```python
from build123d import *

# Parameters (mm, degrees)
BASE_FLANGE1_DEPTH = 390.5
CUT_EXTRUDE2_DEPTH = 419.369827425


# Sheet-metal steps are written as plain solids
with BuildPart() as part:
    # Sketch1 → Base-Flange1 (new, symmetric)
    with BuildSketch(Plane(origin=(0, 0, 0), x_dir=(1, 0, 0), z_dir=(0, 1, 0))):
        with BuildLine():
            Line((9.5, 58), (9.5, 68.0134))
            ThreePointArc((9.5, 68.0134), (10.081861668, 69.418138332), (11.4866, 70))
            Line((11.4866, 70), (37.5134, 70))
            ThreePointArc((37.5134, 70), (38.918138332, 69.418138332), (39.5, 68.0134))
            Line((39.5, 68.0134), (39.5, 23.7366))
            ThreePointArc((39.5, 23.7366), (39.715745145, 23.215745145), (40.2366, 23))
            Line((40.2366, 23), (52.2634, 23))
            ThreePointArc((52.2634, 23), (53.668138332, 22.418138332), (54.25, 21.0134))
            Line((54.25, 21.0134), (54.25, 18))
            Line((54.25, 18), (54.25, -21.0134))
            ThreePointArc((54.25, -21.0134), (53.668138332, -22.418138332), (52.2634, -23))
            Line((52.2634, -23), (40.2366, -23))
            ThreePointArc((40.2366, -23), (39.715745145, -23.215745145), (39.5, -23.7366))
            Line((39.5, -23.7366), (39.5, -68.0134))
            ThreePointArc((39.5, -68.0134), (38.918138332, -69.418138332), (37.5134, -70))
            Line((37.5134, -70), (11.4866, -70))
            ThreePointArc((11.4866, -70), (10.081861668, -69.418138332), (9.5, -68.0134))
            Line((9.5, -68.0134), (9.5, -58))
            Line((9.5, -58), (10.75, -58))
            Line((10.75, -58), (10.75, -68.0134))
            ThreePointArc((10.75, -68.0134), (10.965745145, -68.534254855), (11.4866, -68.75))
            Line((11.4866, -68.75), (37.5134, -68.75))
            ThreePointArc((37.5134, -68.75), (38.034254855, -68.534254855), (38.25, -68.0134))
            Line((38.25, -68.0134), (38.25, -23.7366))
            ThreePointArc((38.25, -23.7366), (38.831861668, -22.331861668), (40.2366, -21.75))
            Line((40.2366, -21.75), (52.2634, -21.75))
            ThreePointArc((52.2634, -21.75), (52.784254855, -21.534254855), (53, -21.0134))
            Line((53, -21.0134), (53, 18))
            Line((53, 18), (53, 21.0134))
            ThreePointArc((53, 21.0134), (52.784254855, 21.534254855), (52.2634, 21.75))
            Line((52.2634, 21.75), (40.2366, 21.75))
            ThreePointArc((40.2366, 21.75), (38.831861668, 22.331861668), (38.25, 23.7366))
            Line((38.25, 23.7366), (38.25, 68.0134))
            ThreePointArc((38.25, 68.0134), (38.034254855, 68.534254855), (37.5134, 68.75))
            Line((37.5134, 68.75), (11.4866, 68.75))
            ThreePointArc((11.4866, 68.75), (10.965745145, 68.534254855), (10.75, 68.0134))
            Line((10.75, 68.0134), (10.75, 58))
            Line((10.75, 58), (9.5, 58))
        make_face()
    extrude(amount=BASE_FLANGE1_DEPTH, both=True)

    # Sketch2 → Cut-Extrude2 (cut, through all)
    with BuildSketch(Plane.XY.offset(70)):
        Polygon((9.5, -390.5), (204.29871247, -195.70128753), (123.087268974, -390.5), align=None)
        Polygon((123.087268974, 390.5), (9.5, 390.5), (204.29871247, 195.70128753), align=None)
    extrude(amount=-CUT_EXTRUDE2_DEPTH, mode=Mode.SUBTRACT)


solid = part.part
```
Model file for the job. Use its own axes, mm. A direction names the side the tool comes from. Give positions to 0.01 mm unless a question says otherwise; leave off trailing zeros. Order: outer loops, then holes, each group sorted by start corner. A loop starts at its lowest first (then second) coordinate and runs counter-clockwise, first axis right, second up.
1) Mould opens along Z. For faces 1 (the flat face through (38.25, 5, 46)), 2 (the flat face through (38.25, 5, -46)), 3 (the flat face through (53.3, 346.7, 0.3)), 4 (the flat face through (25, 5, 70)) say: +Z half, -Z half, draft (parallel to the pull), parting line (faces both ways), or undercut.
2) Wall check: probe 1 along Z at (x, y) = (13, 231); probe 2 along Z at (x, y) = (43, 66.5); probe 3 along X at (y, z) = (-272.5, 30.5). Give the ranges that are in metal, low to high.
3) 3-axis set-ups, long thin cutter, end or side, ignore diameter. For faces 5 (the flat face through (46, 5, 23)), 6 (the flat face through (24, 5, -70)), 7 (the flat face through (25, 5, -68.75)), 8 (the flat face through (39.5, 5, -46)), 9 (the flat face through (53, 5, 0)): which of +Z, -Z, +X, -X, +Y, -Y reach the whole face in a straight line?
4) Saw through at A-A, the plane x = 19.5. Write the cut outline in (y, z).
5) Saw through at B-B, the plane z = 0. Write the cut outline in (x, y), then the cut area to 3 significant figures.
6) Saw through at C-C, the plane z = -32.5. Write the cut outline in (x, y), then the cut area to 3 significant figures.
7) Pin check, flat tips, straight feed: pin 1 (22 mm diameter, centred on y = -155, z = 48.5, fed in from +X); pin 2 (4 mm diameter, centred on y = 312, z = -52, fed in from -X); pin 3 (12.5 mm diameter, centred on y = -173, z = 9.5, fed in from -X). Stop position of each tip, or through.
Computed:
1. face 1: undercut
1. face 2: undercut
1. face 3: draft
1. face 4: +Z half
2. probe 1: z = -70 to -68.75, 68.75 to 70
2. probe 2: z = -23 to -21.75, 21.75 to 23
2. probe 3: x = 38.25 to 39.5
3. face 5: +Z, +X, +Y, -Y
3. face 6: -Z, +X, -X, +Y, -Y
3. face 7: +Y, -Y
3. face 8: -Z, +X, +Y, -Y
3. face 9: -X, +Y, -Y
4. outline: (-380.5, -70) - (380.5, -70) - (380.5, -68.75) - (-380.5, -68.75) - close; (-380.5, 68.75) - (380.5, 68.75) - (380.5, 70) - (-380.5, 70) - close
5. outline: (53, -347) - (54.25, -345.75) - (54.25, 345.75) - (53, 347) - close
5. area: 866 mm2
6. outline: (38.25, -361.75) - (39.5, -360.5) - (39.5, 360.5) - (38.25, 361.75) - close
6. area: 903 mm2
7. pin 1: stops at x = 39.5
7. pin 2: stops at x = 38.25
7. pin 3: stops at x = 53
